Geometry check sheet. Reference: drawing and pictorial views, mm from the part's lowest x, y, z. Give positions to 0.01 mm unless a question says otherwise; leave off trailing zeros. Order: outer loops, then holes, each group sorted by start corner. A loop starts at its lowest first (then second) coordinate and runs counter-clockwise, first axis right, second up.
Item 1: Gauge pin test, flat end, axial feed: P1, Ø9, axis at x = 100, z = 37.5, coming from the +Y side. Record the tip position at first contact, or that the pin passes through.
Item 2: Sectioned sample at A-A on x = 100. Record the boundary of the cut face in (y, z), and give its area (4 significant figures).
Item 3: Material ranges on line 1 along Z through (x, y) = (100, 69); line 2 along X through (y, z) = (71, 37.5), recorded low to high.
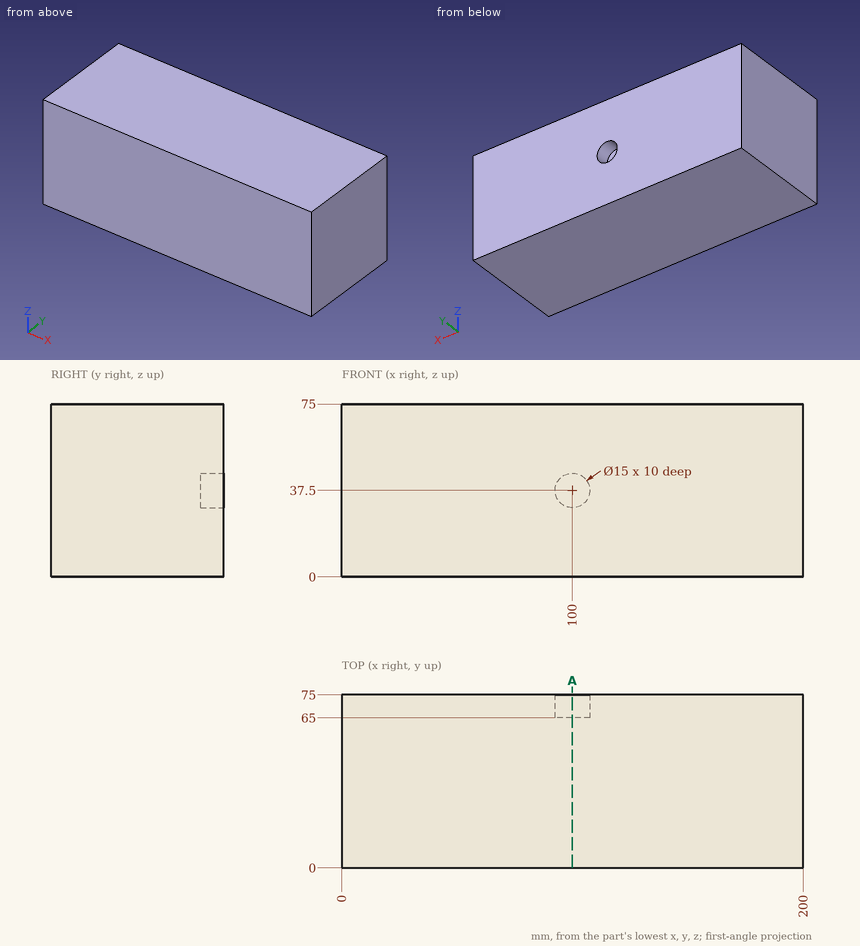
Report:
1. P1: stops at y = 65
2. outline: (0, 0) - (75, 0) - (75, 30) - (65, 30) - (65, 45) - (75, 45) - (75, 75) - (0, 75) - close
2. area: 5,475 mm2
3. line 1: z = 0 to 30, 45 to 75
3. line 2: x = 0 to 92.5, 107.5 to 200
